Read the model definition and answer for the solid it produces. Units are mm, in the model's axes. Round coordinates to 2 decimals unless told otherwise and drop trailing zeros. Order: outer loops, then holes, each group sorted by start corner. A loop starts at its lowest first (then second) coordinate and runs counter-clockwise, first axis right, second up. Notation, with made-up numbers: (34.25, 22.25) - (46.25, 22.25) arc R21 ccw to (46.25, 56.25) - close; hole circle Ø8 at (-24, -3.75). An arc over 180 degrees is marked (long way). Answer as a JSON object with one key per item and string values. Group by question number.
Q1. Given pin 1 Ø6.5 at (y, z) = (-16, 1.5) entering from +X; pin 2 Ø4 at (y, z) = (-15, -1.5) entering from -X; pin 3 Ø6.5 at (y, z) = (-128, -1) entering from +X, each flat-ended and moving along its own axis, determine where each tip first touches the part or whether it passes through.
Q2. A cutting plane is placed at A-A on y = -32. Determine the outline of the cut face in (x, z), and give its area (3 significant figures).
Q3. A cutting plane is placed at D-D on x = 71. Determine the outline of the cut face in (y, z).
Q4. A cutting plane is placed at B-B on z = 3.5. Determine the outline of the cut face in (x, y).
Q5. A cutting plane is placed at C-C on y = -128.5. Determine the outline of the cut face in (x, z), and give its area (3 significant figures).
Q6. Consider line 1 (X direction, y = -40.5, z = 0.5); line 2 (X direction, y = -131.5, z = -2); line 3 (Y direction, x = -2, z = -1). Determine where each line is inside the solid, lowest interval first.
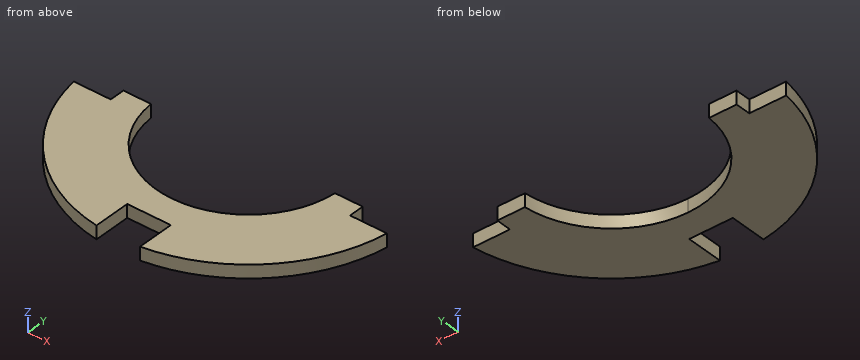
```python
from build123d import *

# Parameters (mm, degrees)
BOSS_EXTRUDE4_DEPTH = 6.35


with BuildPart() as part:
    # Sketch1 → Boss-Extrude4 (new, symmetric)
    with BuildSketch(Plane.XY):
        with BuildLine():
            Line((21, -150.946215587), (21, -115.332))
            Line((21, -115.332), (0, -115.332))
            Line((0, -115.332), (0, -88.9))
            ThreePointArc((0, -88.9), (60.57513929, -65.068137364), (88.672924278, -6.35))
            Line((88.672924278, -6.35), (115.332, -6.35))
            Line((115.332, -6.35), (115.332, -21))
            Line((115.332, -21), (150.946215587, -21))
            ThreePointArc((150.946215587, -21), (107.763073453, -107.763073453), (21, -150.946215587))
        make_face()
    boss_extrude4 = extrude(amount=BOSS_EXTRUDE4_DEPTH, both=True)

    # Mirror1: Boss-Extrude4 across plane
    add(boss_extrude4.mirror(Plane(origin=(0, 0, 0), x_dir=(0, 0, 1), z_dir=(1, 0, 0))))


solid = part.part
```
Result set:
{
 "1": {"pin 1": "stops at x = 115.33", "pin 2": "stops at x = -115.33", "pin 3": "stops at x = 87.54"},
 "2": {"outline": "(-149, -6.35) - (-82.94, -6.35) - (-82.94, 6.35) - (-149, 6.35) - close; (82.94, -6.35) - (149, -6.35) - (149, 6.35) - (82.94, 6.35) - close", "area": "1,680 mm²"},
 "3": {"outline": "(-134.85, -6.35) - (-53.5, -6.35) - (-53.5, 6.35) - (-134.85, 6.35) - close"},
 "4": {"outline": "(-150.95, -21) arc R152.4 ccw to (-21, -150.95) - (-21, -115.33) - (21, -115.33) - (21, -150.95) arc R152.4 ccw to (150.95, -21) - (115.33, -21) - (115.33, -6.35) - (88.67, -6.35) arc R88.9 cw to (-88.67, -6.35) - (-115.33, -6.35) - (-115.33, -21) - close"},
 "5": {"outline": "(-81.94, -6.35) - (-21, -6.35) - (-21, 6.35) - (-81.94, 6.35) - close; (21, -6.35) - (81.94, -6.35) - (81.94, 6.35) - (21, 6.35) - close", "area": "1,550 mm²"},
 "6": {"line 1": "x = -146.92 to -79.14, 79.14 to 146.92", "line 2": "x = -77.03 to -21, 21 to 77.03", "line 3": "y = -115.33 to -88.88"}
}
